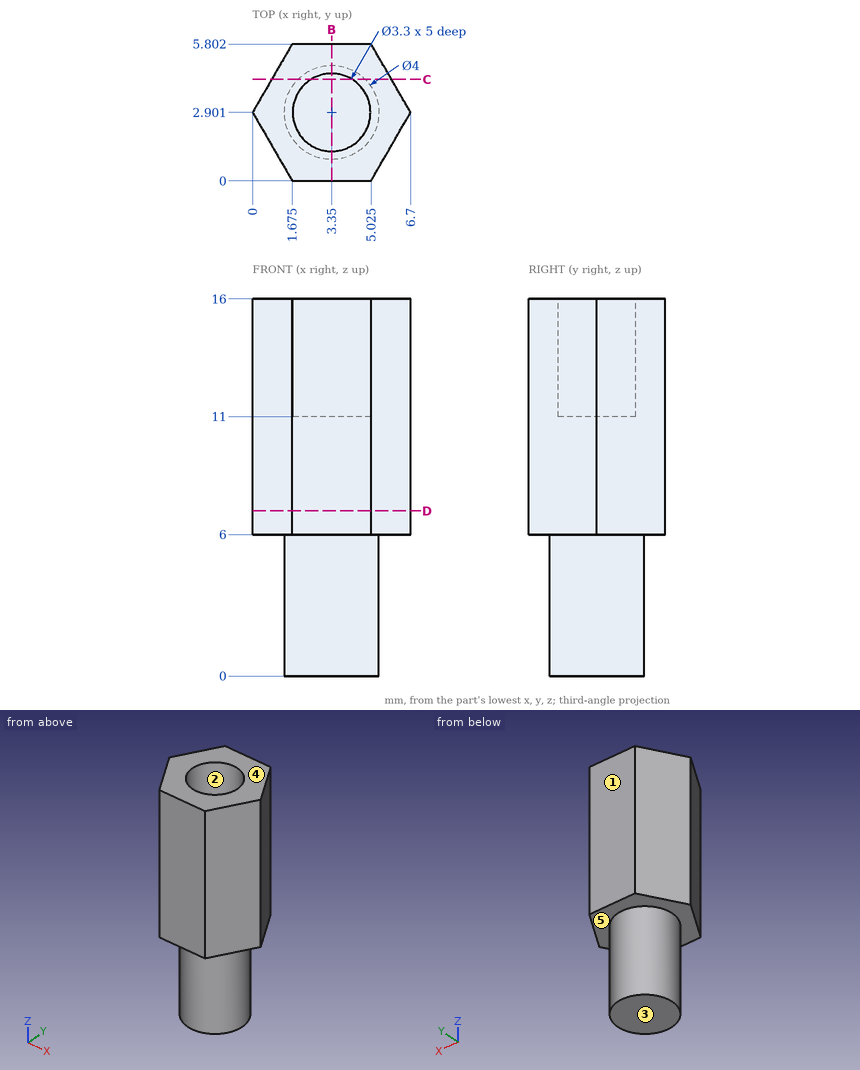
Print and shaded views of the part. All mm, measured from the part's lowest x, y and z. A direction names the side the tool comes from. Give positions to 0.01 mm unless a question says otherwise; leave off trailing zeros. Write each loop counter-clockwise with the first axis right and the second up, starting at its lowest first coordinate (ties: lowest second). Pieces come first, ordered by that corner, then holes. Notation, with made-up numbers: (89, -30.5) -> (145, -30.5) arc R11 cw to (145, -17.5) -> close; hole circle Ø11 at (-27.5, 47). An arc over 180 degrees is marked (long way). Write item = value, one per line.
(1) Mould opens along Y. For the marked faces 1, 2 and 3 say: released by +Y, released by -Y, zero draft, split by the parting line, or undercut.
Determined:
face_1 = released by +Y
face_2 = undercut
face_3 = zero draft
(2) Slice it at B-B, the plane x = 3.35. Give the cut face in (y, z).
Determined:
outline = (0, 6) -> (0.9, 6) -> (0.9, 0) -> (4.9, 0) -> (4.9, 6) -> (5.8, 6) -> (5.8, 16) -> (4.55, 16) -> (4.55, 11) -> (1.25, 11) -> (1.25, 16) -> (0, 16) -> close
(3) Probe line 1 along Y through (x, z) = (3.35, 12.35); line 2 along Y through (x, z) = (2.5, 14.25) (1 decimal); line 3 along Z through (x, y) = (0.5, 2.75). List the from-to ranges inside material, lowest first.
Determined:
line_1 = 0 to 1.25, 4.55 to 5.8
line_2 = 0 to 1.5, 4.3 to 5.8
line_3 = 6 to 16
(4) Slice it at C-C, the plane y = 4.3. Give the cut face in (x, z) (1 decimal).
Determined:
outline = (0.8, 6) -> (1.9, 6) -> (1.9, 0) -> (4.8, 0) -> (4.8, 6) -> (5.9, 6) -> (5.9, 16) -> (4.2, 16) -> (4.2, 11) -> (2.5, 11) -> (2.5, 16) -> (0.8, 16) -> close
(5) Flat gauge pins, fed straight in: P1, Ø3, axis at x = 5, z = 3.5, coming from the -Y side; P2, Ø2, axis at x = 3.35, y = 2.9, coming from the +Z side. Where does each tip first touch, or does it go through?
Determined:
P1 = 0.91
P2 = 11
(6) Tool access for the marked faces 4 and 5: list every direction of +Z, -Z, +X, -X, +Y, -Y with a clear straight run to the whole face (end or side of a thin tool).
Determined:
face_4 = +Z, +X, -X, +Y, -Y
face_5 = -Z
(7) Slice it at D-D, the plane z = 7. Give the cut face in (x, y) (1 decimal).
Determined:
outline = (0, 2.9) -> (1.7, 0) -> (5, 0) -> (6.7, 2.9) -> (5, 5.8) -> (1.7, 5.8) -> close
